Job drawing, mm, ordinate dimensions from the low corner. One solid piece. Give positions to 0.01 mm unless a question says otherwise; leave off trailing zeros. Loops run counter-clockwise (first coordinate to the right, second up) from the corner with the lowest first, then second, coordinate; pieces in that order, holes last.
Item 1: Saw through at B-B on x = 305. Give the cut face in (y, z).
Item 2: Saw through at A-A on y = 8. Give the cut face in (x, z).
Item 3: Drop flat-ended pins along their axis: P1, Ø22, axis at x = 188.5, y = 25, coming from the +Z side; P2, Ø10, axis at x = 273, z = 374.5, coming from the -Y side; P3, Ø16, axis at x = 107, z = 197.5, coming from the +Y side. Give the stop position or say it passes through.
Item 4: Probe probe 1 along Z at (x, y) = (379, 29); probe 2 along X at (y, z) = (8, 279); probe 3 along Y at (x, z) = (187, 100.5). List the from-to ranges inside material, lowest first.
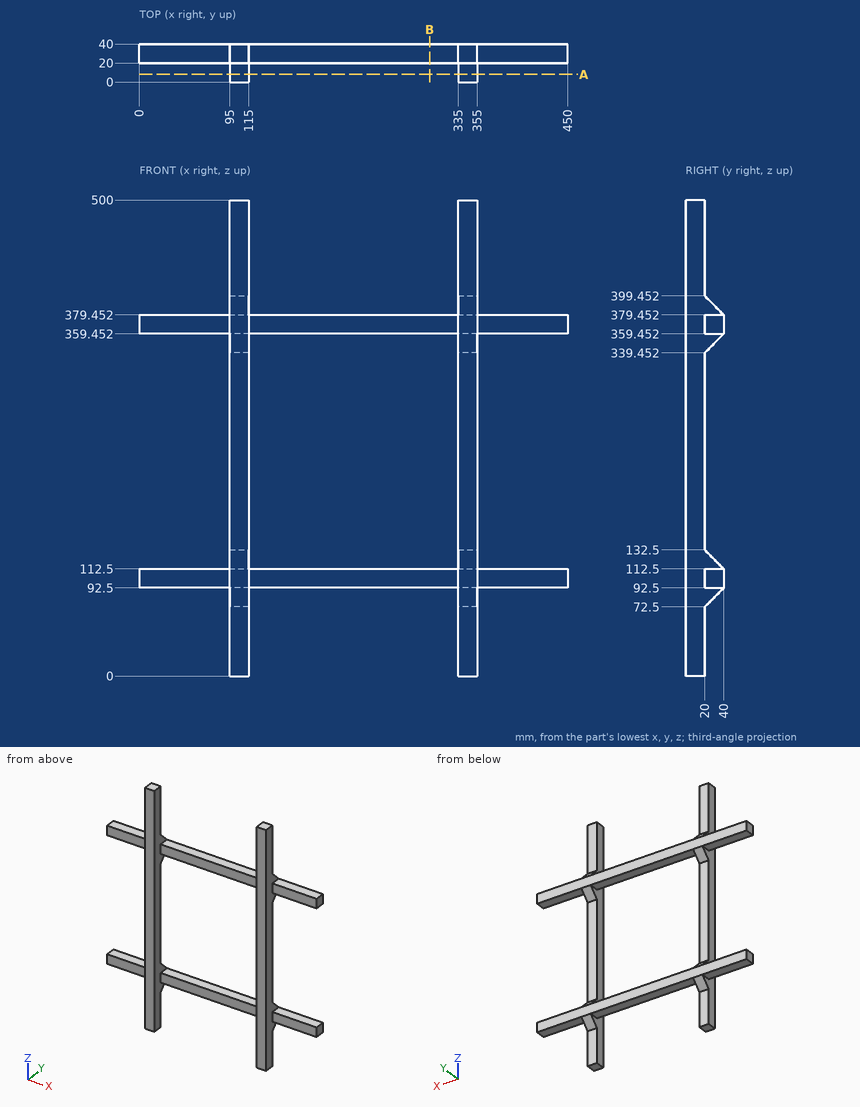
Results below:
1. outline: (20, 92.5) - (40, 92.5) - (40, 112.5) - (20, 112.5) - close; (20, 359.45) - (40, 359.45) - (40, 379.45) - (20, 379.45) - close
2. outline: (95, 0) - (115, 0) - (115, 500) - (95, 500) - close; (335, 0) - (355, 0) - (355, 500) - (335, 500) - close
3. P1: stops at z = 379.45
3. P2: stops at y = 20
3. P3: stops at y = 20
4. probe 1: z = 92.5 to 112.5, 359.45 to 379.45
4. probe 2: x = 95 to 115, 335 to 355
4. probe 3: y = 20 to 40
